For this review, use the dimensioned drawing (mm, ordinates from the lowest corner) and the shaded views. A direction names the side the tool comes from. Coordinates: 2 decimals unless noted, no trailing zeros. Write each loop counter-clockwise with the first axis right and the second up, starting at its lowest first coordinate (ties: lowest second). Pieces come first, ordered by that corner, then holes. Notation, with made-up numbers: (-24.75, 0) -> (-0.75, 0) arc R10 ccw to (-0.75, 14) -> close; hole circle Ø6 at (36.5, -39.5). An arc over 180 degrees is marked (long way). Put each result on its own line as item: value. Start each with the question number.
Item 1: The part is to be moulded in two halves that separate along X. For the marked faces 3, 4 and 5, say which applies: +X half, -X half, draft (parallel to the pull), parting line (faces both ways), or undercut.
Item 2: Consider section A-A on y = 7. Give the boundary of the cut face in (x, z).
Item 3: To check wall thickness, follow L1, parallel to X at y = 23.5, z = 16; L2, parallel to Y at x = 23, z = 8. State the ranges of each line that lie inside material, in increasing order.
Item 4: For the marked faces 1 and 2, list the 3-axis set-ups (+Z, -Z, +X, -X, +Y, -Y) from which the entire face can be reached by the end or side of a thin tool; tool diameter is ignored.
Item 5: Insertion check: P1, Ø6, axis at x = 10, z = 11, coming from the +Y side. The pin has a flat end and moves straight along its axis. Give the tip position at first contact, or say it passes through.
Item 6: Consider section B-B on z = 12. Give the boundary of the cut face in (x, y), and give its area (3 significant figures).
Item 7: Consider section C-C on x = 31. Give the boundary of the cut face in (y, z), and give its area (3 significant figures).
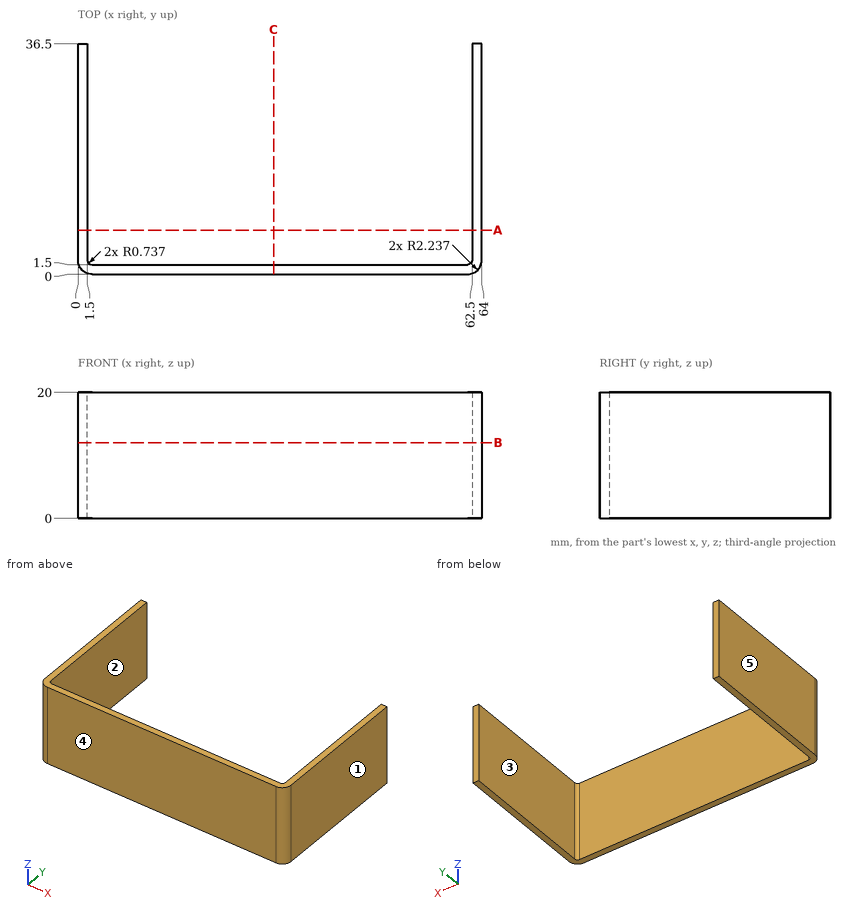
Return value:
1. face 3: undercut
1. face 4: draft
1. face 5: -X half
2. outline: (0, 0) -> (1.5, 0) -> (1.5, 20) -> (0, 20) -> close; (62.5, 0) -> (64, 0) -> (64, 20) -> (62.5, 20) -> close
3. L1: 0 to 1.5, 62.5 to 64
3. L2: 0 to 1.5
4. face 1: +Z, -Z, +X, +Y, -Y
4. face 2: +Z, -Z, +Y
5. P1: y = 1.5
6. outline: (0, 2.24) arc R2.24 ccw to (2.24, 0) -> (61.76, 0) arc R2.24 ccw to (64, 2.24) -> (64, 36.5) -> (62.5, 36.5) -> (62.5, 2.24) arc R0.74 cw to (61.76, 1.5) -> (2.24, 1.5) arc R0.74 cw to (1.5, 2.24) -> (1.5, 36.5) -> (0, 36.5) -> close
6. area: 199 mm^2
7. outline: (0, 0) -> (1.5, 0) -> (1.5, 20) -> (0, 20) -> close
7. area: 30.0 mm^2
